```python
from build123d import *


with BuildPart() as part:
    # Sketch1 → Loft2 section 0
    with BuildSketch(Plane.XY):
        with BuildLine():
            Line((-14.749435925, 1.579146396), (-13.769485327, 2.95855378))
            ThreePointArc((-13.769485327, 2.95855378), (-13.585390404, 3.574613199), (-13.814433877, 4.175412031))
            add(Edge.make_bspline(
                [(-13.814433877, 4.175412031), (-14.417527952, 4.903873153), (-17.567781248, 7.791225194), (-22.06162275, 8.841915434), (-25.318719368, 8.741869045)],
                knots=[0.056598746, 0.056598746, 0.056598746, 0.056598746, 0.264504946, 1, 1, 1, 1], degree=3))
            Line((-25.318719368, 8.741869045), (-27.784310983, 8.741869045))
            add(Edge.make_bspline(
                [(-29.323229714, 9.211162218), (-28.911734347, 8.939401458), (-28.272403474, 8.743384076), (-27.784310983, 8.741869045)],
                knots=[0.586596628, 0.586596628, 0.586596628, 0.586596628, 1, 1, 1, 1], degree=3))
            ThreePointArc((-29.323229714, 9.211162218), (-29.747065132, 10.268151444), (-28.906559125, 11.036534382))
            ThreePointArc((-28.906559125, 11.036534382), (-24.721817141, 17.633736944), (-31.933702711, 20.637709922))
            ThreePointArc((-31.933702711, 20.637709922), (-32.573936169, 20.54323377), (-33.137949221, 20.860588307))
            Line((-33.137949221, 20.860588307), (-33.224181658, 20.957186689))
            ThreePointArc((-33.224181658, 20.957186689), (-33.468334903, 21.763124392), (-33.010324904, 22.46978784))
            ThreePointArc((-33.010324904, 22.46978784), (-28.072687528, 23.43565364), (-23.764465571, 20.837118829))
            ThreePointArc((-23.764465571, 20.837118829), (-23.196744837, 20.168506773), (-22.572618747, 19.552215012))
            Line((-22.572618747, 19.552215012), (-7.145865193, 5.601063972))
            ThreePointArc((-7.145865193, 5.601063972), (-4.032245088, 3.686045747), (-0.43842089, 3.017949499))
            Line((-0.43842089, 3.017949499), (0.43842089, 3.017949499))
            ThreePointArc((0.43842089, 3.017949499), (4.032245088, 3.686045747), (7.145865193, 5.601063972))
            Line((7.145865193, 5.601063972), (22.572618747, 19.552215012))
            ThreePointArc((22.572618747, 19.552215012), (23.196744837, 20.168506773), (23.764465571, 20.837118829))
            ThreePointArc((23.764465571, 20.837118829), (28.072687528, 23.43565364), (33.010324904, 22.46978784))
            ThreePointArc((33.010324904, 22.46978784), (33.468334903, 21.763124392), (33.224181658, 20.957186689))
            Line((33.224181658, 20.957186689), (33.137949221, 20.860588307))
            ThreePointArc((33.137949221, 20.860588307), (32.573936169, 20.54323377), (31.933702711, 20.637709922))
            ThreePointArc((31.933702711, 20.637709922), (24.721817141, 17.633736944), (28.906559125, 11.036534382))
            ThreePointArc((28.906559125, 11.036534382), (29.747065132, 10.268151444), (29.323229714, 9.211162218))
            add(Edge.make_bspline(
                [(29.323229714, 9.211162218), (28.911734347, 8.939401458), (28.272403474, 8.743384076), (27.784310983, 8.741869045)],
                knots=[0.586596628, 0.586596628, 0.586596628, 0.586596628, 1, 1, 1, 1], degree=3))
            Line((27.784310983, 8.741869045), (25.318719368, 8.741869045))
            add(Edge.make_bspline(
                [(13.814433877, 4.175412031), (14.417527952, 4.903873153), (17.567781248, 7.791225194), (22.06162275, 8.841915434), (25.318719368, 8.741869045)],
                knots=[0.056598746, 0.056598746, 0.056598746, 0.056598746, 0.264504946, 1, 1, 1, 1], degree=3))
            ThreePointArc((13.814433877, 4.175412031), (13.585390404, 3.574613199), (13.769485327, 2.95855378))
            Line((13.769485327, 2.95855378), (14.749435925, 1.579146396))
            ThreePointArc((14.749435925, 1.579146396), (14.822791679, 0.541276988), (13.934212365, 0))
            Line((13.934212365, 0), (-13.934212365, 0))
            ThreePointArc((-13.934212365, 0), (-14.822791679, 0.541276988), (-14.749435925, 1.579146396))
        make_face()
    # Sketch7 → Loft2 section 1
    with BuildSketch(Plane.XY.offset(10)):
        with BuildLine():
            Line((-14.749435925, 1.579146396), (-13.769485327, 2.95855378))
            ThreePointArc((-13.769485327, 2.95855378), (-13.585390404, 3.574613199), (-13.814433877, 4.175412031))
            add(Edge.make_bspline(
                [(-13.814433877, 4.175412031), (-14.417527952, 4.903873153), (-17.567781248, 7.791225194), (-22.06162275, 8.841915434), (-25.318719368, 8.741869045)],
                knots=[0.056598746, 0.056598746, 0.056598746, 0.056598746, 0.264504946, 1, 1, 1, 1], degree=3))
            Line((-25.318719368, 8.741869045), (-27.784310983, 8.741869045))
            add(Edge.make_bspline(
                [(-29.323229714, 9.211162218), (-28.911734347, 8.939401458), (-28.272403474, 8.743384076), (-27.784310983, 8.741869045)],
                knots=[0.586596628, 0.586596628, 0.586596628, 0.586596628, 1, 1, 1, 1], degree=3))
            ThreePointArc((-29.323229714, 9.211162218), (-29.747065132, 10.268151444), (-28.906559125, 11.036534382))
            ThreePointArc((-28.906559125, 11.036534382), (-24.721817141, 17.633736944), (-31.933702711, 20.637709922))
            ThreePointArc((-31.933702711, 20.637709922), (-32.573936169, 20.54323377), (-33.137949221, 20.860588307))
            Line((-33.137949221, 20.860588307), (-33.224181658, 20.957186689))
            ThreePointArc((-33.224181658, 20.957186689), (-33.468334903, 21.763124392), (-33.010324904, 22.46978784))
            ThreePointArc((-33.010324904, 22.46978784), (-28.072687528, 23.43565364), (-23.764465571, 20.837118829))
            ThreePointArc((-23.764465571, 20.837118829), (-23.196744837, 20.168506773), (-22.572618747, 19.552215012))
            Line((-22.572618747, 19.552215012), (-7.145865193, 5.601063972))
            ThreePointArc((-7.145865193, 5.601063972), (-4.032245088, 3.686045747), (-0.43842089, 3.017949499))
            Line((-0.43842089, 3.017949499), (0.43842089, 3.017949499))
            ThreePointArc((0.43842089, 3.017949499), (4.032245088, 3.686045747), (7.145865193, 5.601063972))
            Line((7.145865193, 5.601063972), (22.572618747, 19.552215012))
            ThreePointArc((22.572618747, 19.552215012), (23.196744837, 20.168506773), (23.764465571, 20.837118829))
            ThreePointArc((23.764465571, 20.837118829), (28.072687528, 23.43565364), (33.010324904, 22.46978784))
            ThreePointArc((33.010324904, 22.46978784), (33.468334903, 21.763124392), (33.224181658, 20.957186689))
            Line((33.224181658, 20.957186689), (33.137949221, 20.860588307))
            ThreePointArc((33.137949221, 20.860588307), (32.573936169, 20.54323377), (31.933702711, 20.637709922))
            ThreePointArc((31.933702711, 20.637709922), (24.721817141, 17.633736944), (28.906559125, 11.036534382))
            ThreePointArc((28.906559125, 11.036534382), (29.747065132, 10.268151444), (29.323229714, 9.211162218))
            add(Edge.make_bspline(
                [(29.323229714, 9.211162218), (28.911734347, 8.939401458), (28.272403474, 8.743384076), (27.784310983, 8.741869045)],
                knots=[0.586596628, 0.586596628, 0.586596628, 0.586596628, 1, 1, 1, 1], degree=3))
            Line((27.784310983, 8.741869045), (25.318719368, 8.741869045))
            add(Edge.make_bspline(
                [(13.814433877, 4.175412031), (14.417527952, 4.903873153), (17.567781248, 7.791225194), (22.06162275, 8.841915434), (25.318719368, 8.741869045)],
                knots=[0.056598746, 0.056598746, 0.056598746, 0.056598746, 0.264504946, 1, 1, 1, 1], degree=3))
            ThreePointArc((13.814433877, 4.175412031), (13.585390404, 3.574613199), (13.769485327, 2.95855378))
            Line((13.769485327, 2.95855378), (14.749435925, 1.579146396))
            ThreePointArc((14.749435925, 1.579146396), (14.822791679, 0.541276988), (13.934212365, 0))
            Line((13.934212365, 0), (-13.934212365, 0))
            ThreePointArc((-13.934212365, 0), (-14.822791679, 0.541276988), (-14.749435925, 1.579146396))
        make_face()
    loft()


solid = part.part
```
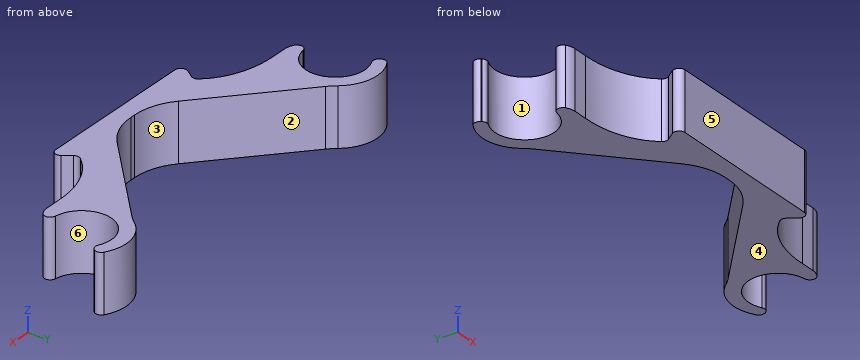
Could you check a few things on this model? Use its own coordinates, in mm. Face numbers are marked on the shaded views. A direction names the side the tool comes from. Round coordinates to 2 decimals unless told otherwise and drop trailing zeros. Order: outer loops, then holes, each group sorted by start corner. A loop starts at its lowest first (then second) coordinate and runs counter-clockwise, first axis right, second up. Notation, with made-up numbers: M 61,-28.5 L 120,-28.5 A23 ccw 120,3.5 Z; hole C 65.5,4.25 d6. An arc over 180 degrees is marked long. One line per question, with ' | ' between items. Start each with the question number.
(1) Thinking about a two-plate mould opening in Y: for the marked faces 3, 4, 5 and 6, which applies, +Y half, -Y half, draft (parallel to the pull), parting line (faces both ways), or undercut?
(2) Suppose I cut it at B-B on y = 16.5. List the corners of the cut face in (x, z) for me.
(3) For P1, Ø6, axis at x = -5, z = 8.5, coming from the +Y side; P2, Ø1, axis at x = 22.5, z = 6, coming from the +Y side; P3, Ø2, axis at x = 17.5, y = 15, coming from the +Z side; P4, Ø1, axis at x = 0, z = 6, coming from the +Y side, each with a flat end and sliding along its axis, tell me the tip position at first contact or that it passes through.
(4) Please list where these lines run through material, in increasing order: line 1 along X through (y, z) = (18.25, 3.75); line 2 along Y through (x, z) = (25, 7); line 3 along X through (y, z) = (13, 4.5).
(5) Suppose I cut it at C-C on x = 11.5. List the corners of the cut face in (y, z) for me.
(6) Suppose I cut it at A-A on y = 12.5. List the corners of the cut face in (x, z) for me.
(7) For the marked faces 1 and 2, which set-ups out of +Z, -Z, +X, -X, +Y, -Y let a thin tool reach every point of the face, with its end or its side?
Geometry results:
1) face 3: +Y half | face 4: draft | face 5: -Y half | face 6: undercut
2) outline: M -24.5,0 L -19.2,0 L -19.2,10 L -24.5,10 Z; M 19.2,0 L 24.5,0 L 24.5,10 L 19.2,10 Z
3) P1: y = 6.37 | P2: y = 19.96 | P3: z = 10 | P4: y = 3.02
4) line 1: -24.96 to -21.13, 21.13 to 24.96 | line 2: 8.75 to 13.86, 18.33 to 22.07 | line 3: -25.53 to -15.33, 15.33 to 25.53
5) outline: M 0,0 L 9.54,0 L 9.54,10 L 0,10 Z
6) outline: M -25.97,0 L -14.77,0 L -14.77,10 L -25.97,10 Z; M 14.77,0 L 25.97,0 L 25.97,10 L 14.77,10 Z
7) face 1: +Z, -Z | face 2: +Z, -Z, +Y
